Autodesk Inventor part; units mm, degrees
ref_plane "YZ Plane" through (0, 0, 0) normal (1, 0, 0) x (0, 1, 0)
ref_plane "XZ Plane" through (0, 0, 0) normal (0, 1, 0) x (-1, 0, 0)
ref_plane "XY Plane" through (0, 0, 0) normal (0, 0, 1) x (1, 0, 0)
sketch "Sketch1" plane through (0, 0, 0) normal (0, 0, 1) x (1, 0, 0)
  line L0 (0, 0) -> (0, 38.1)
  line L1 (0, 38.1) -> (393.7, 38.1)
  line L2 (393.7, 38.1) -> (393.7, 0)
  line L3 (393.7, 0) -> (0, 0)
  circle A0 centre (127, 19.05) radius 18.542
  circle A1 centre (222.25, 19.05) radius 18.542
  circle A2 centre (170.942, 19.05) radius 1.778
  circle A3 centre (266.192, 19.05) radius 1.778
  line L4 (151.003, 19.05) -> (151.003, 26.0604)
  circle A4 centre (102.997, 12.0396) radius 1.7526
  circle A5 centre (102.997, 26.0604) radius 1.7526
  circle A6 centre (151.003, 26.0604) radius 1.7526
  circle A7 centre (151.003, 12.0396) radius 1.7526
  line L5 (151.003, 19.05) -> (127, 19.05)
  circle A8 centre (246.253, 26.0604) radius 1.7526
  circle A9 centre (246.253, 12.0396) radius 1.7526
  circle A10 centre (198.247, 12.0396) radius 1.7526
  circle A11 centre (198.247, 26.0604) radius 1.7526
  circle A12 centre (50.8, 12.7) radius 6.35
  circle A13 centre (342.9, 12.7) radius 6.35
  dimension "d0" = 38.1
  dimension "d1" = 393.7
  dimension "d3" = 37.084
  dimension "d5" = 37.084
  dimension "d10" = 3.556
  dimension "d11" = 3.556
  dimension "d24" = 7.0104
  dimension "d28" = 3.5052
  dimension "d29" = 3.5052
  dimension "d30" = 3.5052
  dimension "d31" = 24.003
  dimension "d38" = 3.5052
  dimension "d39" = 3.5052
  dimension "d40" = 3.5052
  dimension "d41" = 3.5052
  dimension "d48" = 12.7
  dimension "d50" = 12.7
extrude "Extrusion1" add sketch "Sketch1" along normal blind 6.35 contours L0 L1 L2 L3 | A6 | A2 | A3 | A4 | A5 | A7 | A8 | A9 | A10 | A11 | A12 | A13
hole "Hole1" at (170.942, 19.05, 0) at (266.192, 19.05, 0) direction (0, 0, 1) diameter 3.556 end through all
chamfer "Chamfer1" distance 3.175 angle 45 2 edges at (170.942, 17.272, 6.35) (266.192, 17.272, 6.35)
extrude "Extrusion2" cut sketch "Sketch1" along normal blind 6.35 contours A8 | A9
extrude "Extrusion3" cut sketch "Sketch1" along normal blind 6.35 contours A6 | A4 | A5 | A7 | A10 | A11
extrude "Extrusion4" cut sketch "Sketch1" along normal blind 25.4 contours A12 | A13
chamfer "Chamfer2" distance 12.7 angle 45 1 edges at (0, 0, 3.175)
chamfer "Chamfer3" distance 12.7 angle 45 1 edges at (393.7, 0, 3.175)
properties part number "Drive Train - Smallest Model"
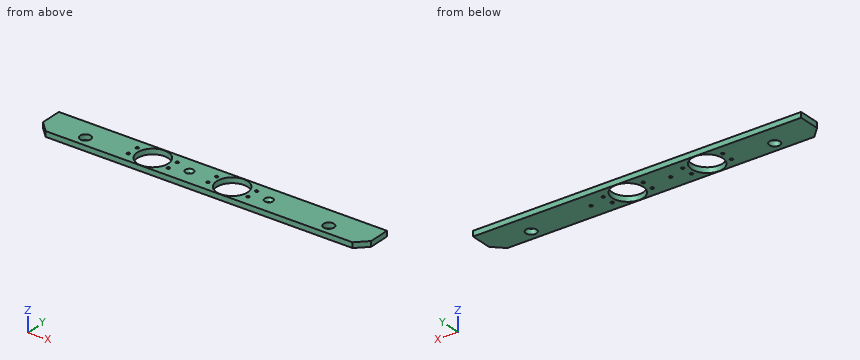
Part model, mm, in its own coordinate system. Round coordinates to 2 decimals unless told otherwise and drop trailing zeros. Loops run counter-clockwise (first coordinate to the right, second up) from the corner with the lowest first, then second, coordinate; pieces in that order, holes last.
1. Slice it at D-D (x = 342.9). Give the cut face in (y, z), and give its area (3 significant figures).
Solutions:
outline: (0, 0) - (6.35, 0) - (6.35, 6.35) - (0, 6.35) - close; (19.05, 0) - (38.1, 0) - (38.1, 6.35) - (19.05, 6.35) - close
area: 161 mm2
2. Slice it at A-A (x = 127). Give the cut face in (y, z).
Solutions:
outline: (0, 0) - (0.51, 0) - (0.51, 6.35) - (0, 6.35) - close; (37.59, 0) - (38.1, 0) - (38.1, 6.35) - (37.59, 6.35) - close
3. Slice it at C-C (z = 4.75). Count the separate pieces of the cut face and the enclosed holes in it, and give its area (3 significant figures).
Solutions:
separate pieces: 1
enclosed holes: 14
area: 12,300 mm2
4. Drill centre lines: line 1 along Y through (x, z) = (127, 2.25); line 2 along X through (y, z) = (7.5, 1.25); line 3 along X through (y, z) = (4.5, 3.5). Where is each one in solid material? Low to high.
Solutions:
line 1: y = 0 to 0.51, 37.59 to 38.1
line 2: x = 5.2 to 47.16, 54.44 to 112.49, 141.51 to 207.74, 236.76 to 339.26, 346.54 to 388.5
line 3: x = 8.2 to 115.51, 138.49 to 210.76, 233.74 to 385.5
5. Slice it at B-B (y = 32). Give the cut face in (x, z).
Solutions:
outline: (0, 0) - (113.73, 0) - (113.73, 6.35) - (0, 6.35) - close; (140.27, 0) - (208.98, 0) - (208.98, 6.35) - (140.27, 6.35) - close; (235.52, 0) - (393.7, 0) - (393.7, 6.35) - (235.52, 6.35) - close
